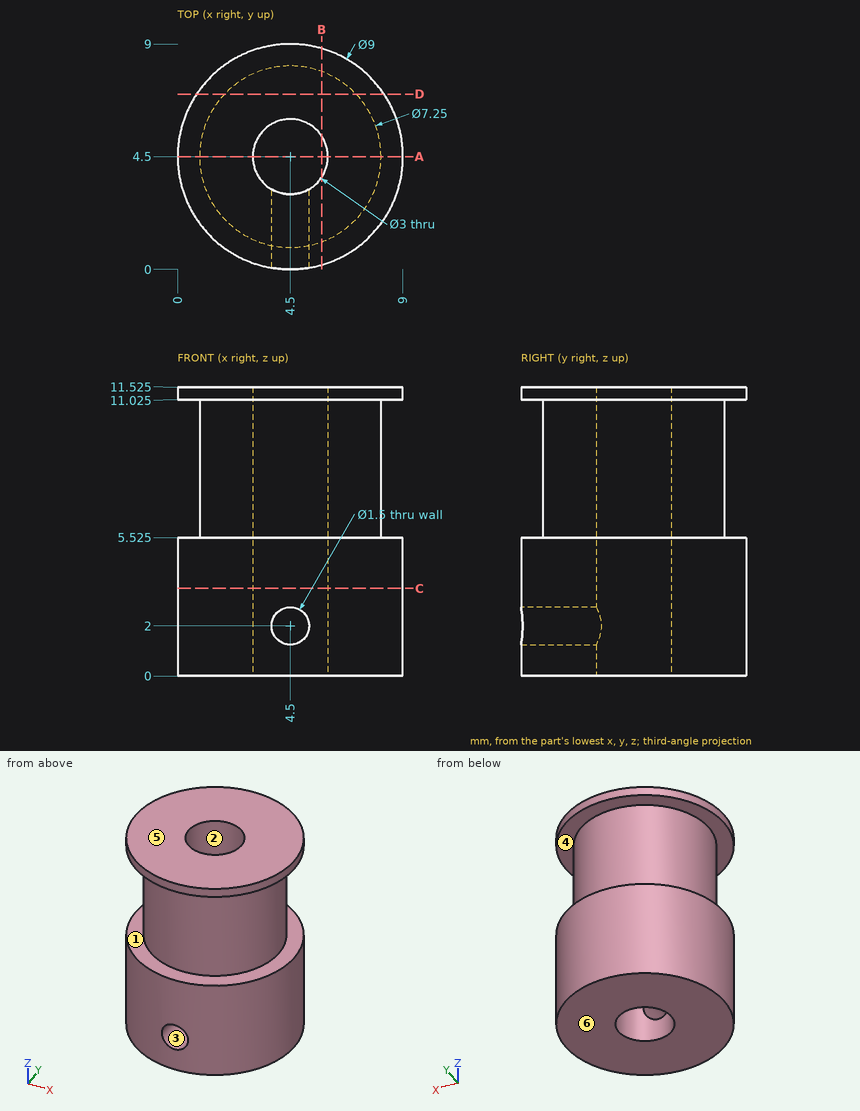
Answer from the drawing. Dimensions are ordinates in mm from the lowest x, y and z of the part. A direction names the side the tool comes from. Give positions to 0.01 mm unless a question says otherwise; leave off trailing zeros. Write each loop counter-clockwise with the first axis right and the second up, starting at its lowest first coordinate (ties: lowest second). Pieces come first, ordered by that corner, then holes. Notation, with made-up numbers: M 52,28 L 100,28 A24 cw 100,53 Z; hole C 40,69 d6. An arc over 180 degrees is marked long. Answer as CSV lines item,"result".
Q1. Find the intervals of material crossed by probe 1 along Y at (x, z) = (4.5, 6) (3 decimals); probe 2 along Y at (x, z) = (4.5, 4); probe 3 along X at (y, z) = (3.25, 6), in increasing order. Write a range as [from, to].
A:
probe 1,"y = [0.875, 3], [6, 8.125]"
probe 2,"y = [0, 3], [6, 9]"
probe 3,"x = [1.1, 3.67], [5.33, 7.9]"
Q2. A cutting plane is placed at C-C on z = 3.5. Write down the section's boundary in (x, y), plus the area to 3 significant figures.
A:
outline,"C 4.5,4.5 d9; hole C 4.5,4.5 d3"
area,"56.5 mm²"
Q3. A cutting plane is placed at D-D on y = 7. Write down the section's boundary in (x, z) (3 decimals).
A:
outline,"M 0.758,0 L 8.242,0 L 8.242,5.525 L 7.125,5.525 L 7.125,11.025 L 8.242,11.025 L 8.242,11.525 L 0.758,11.525 L 0.758,11.025 L 1.875,11.025 L 1.875,5.525 L 0.758,5.525 Z"
Q4. A cutting plane is placed at A-A on y = 4.5. Write down the section's boundary in (x, z) (3 decimals), plus the area to 3 significant figures.
A:
outline,"M 0,0 L 3,0 L 3,11.525 L 0,11.525 L 0,11.025 L 0.875,11.025 L 0.875,5.525 L 0,5.525 Z; M 6,0 L 9,0 L 9,5.525 L 8.125,5.525 L 8.125,11.025 L 9,11.025 L 9,11.525 L 6,11.525 Z"
area,"59.5 mm²"
Q5. The mould has two halves that part along Z. Classify the marked faces 4, 5 and 6: +Z half, -Z half, draft (parallel to the pull), parting line (faces both ways), or undercut.
A:
face 4,"undercut"
face 5,"+Z half"
face 6,"-Z half"
Q6. A cutting plane is placed at B-B on x = 5.75. Write down the section's boundary in (y, z) (3 decimals).
A:
outline,"M 0.177,0 L 3.671,0 L 3.671,11.525 L 0.177,11.525 L 0.177,11.025 L 1.097,11.025 L 1.097,5.525 L 0.177,5.525 Z; M 5.329,0 L 8.823,0 L 8.823,5.525 L 7.903,5.525 L 7.903,11.025 L 8.823,11.025 L 8.823,11.525 L 5.329,11.525 Z"
Q7. A tool of negligible diameter and unlimited length cuts with its end or side. For the marked faces 1, 2 and 3, from which of +Z, -Z, +X, -X, +Y, -Y can it reach the whole face along a straight path? Write none if from no direction.
A:
face 1,"none"
face 2,"+Z, -Z"
face 3,"-Y"
Q8. Given P1, Ø2.5, axis at x = 4.5, y = 4.5, coming from the -Z side; P2, Ø1.5, axis at y = 1, z = 3, coming from the -X side, each flat-ended and moving along its own axis, determine where each tip first touches the part or whether it passes through.
A:
P1,"passes through"
P2,"stops at x = 0.94"
